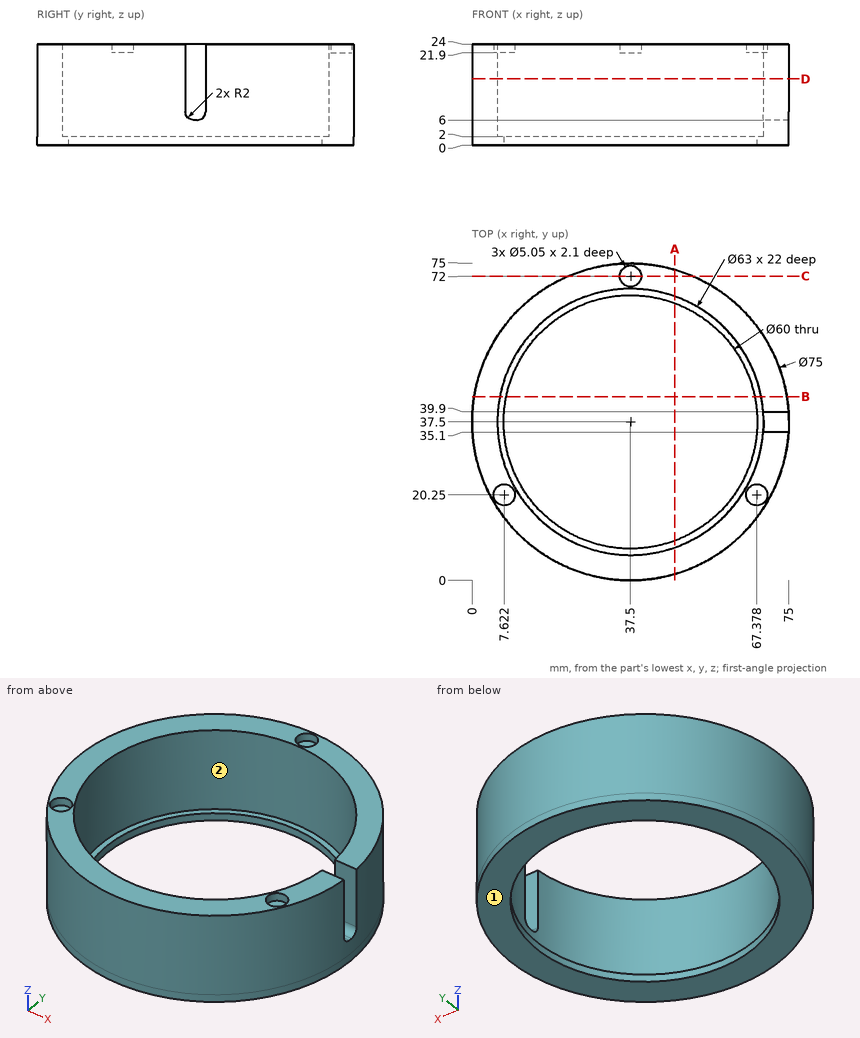
Could you check a few things on this drawing? It's one solid part, dimensions in mm from its lowest x, y, z. Coordinates: 2 decimals unless noted, no trailing zeros. Loops run counter-clockwise (first coordinate to the right, second up) from the corner with the lowest first, then second, coordinate; pieces in that order, holes last. Notation, with made-up numbers: (-30, 6) - (-18, 6) arc R32 cw to (-18, 37) - close; hole circle Ø2 at (11, 27.5). An arc over 180 degrees is marked (long way). Answer as a JSON object with one key per item and string values. Group by question number.
Item 1: If we section it at A-A (x = 48): List the corners of the cut face in (y, z) for me.
Item 2: If we mould it in two halves opening along Y, with no side actions, what happens to the marked faces 1 and 2? For each: released by +Y, released by -Y, zero draft, split by the parting line, or undercut.
Item 3: For pin 1 (0.9 mm diameter, centred on x = 72.5, y = 37.5, fed in from +Z); pin 2 (5 mm diameter, centred on x = 40.5, z = 14, fed in from -Y); pin 3 (6.5 mm diameter, centred on x = 73.5, z = 19, fed in from +Y); pin 4 (5 mm diameter, centred on x = 43.5, y = 12.5, fed in from -Z), each with a flat end and sliding along its axis, tell me the tip position at first contact or that it passes through.
Item 4: If we section it at D-D (z = 15.75): List the corners of the cut face in (x, y) for me, plus the area to 3 significant figures.
Item 5: If we section it at B-B (y = 43.5): List the corners of the cut face in (x, z) for me, plus the area to 3 significant figures.
Item 6: If I drill on L1, parallel to Y at x = 37.5, z = 17.5; L2, parallel to X at y = 20.25, z = 22.65; L3, parallel to Z at x = 66.5, y = 29.5, over which ranges is the centre line in solid material (lowest first)? Write a range as from..to.
Item 7: If we section it at C-C (y = 72): List the corners of the cut face in (x, z) for me (3 decimals).
Returned:
{
 "1": {"outline": "(1.5, 0) - (9.4, 0) - (9.4, 2) - (7.8, 2) - (7.8, 24) - (1.5, 24) - close; (65.6, 0) - (73.5, 0) - (73.5, 24) - (67.2, 24) - (67.2, 2) - (65.6, 2) - close"},
 "2": {"face 1": "zero draft", "face 2": "undercut"},
 "3": {"pin 1": "stops at z = 6", "pin 2": "stops at y = 0", "pin 3": "stops at y = 55.77", "pin 4": "passes through"},
 "4": {"outline": "(68.91, 35.1) arc R31.5 cw (long way) to (68.91, 39.9) - (74.92, 39.9) arc R37.5 ccw (long way) to (74.92, 35.1) - close", "area": "1,270 mm²"},
 "5": {"outline": "(0.48, 0) - (8.11, 0) - (8.11, 2) - (6.58, 2) - (6.58, 24) - (0.48, 24) - close; (66.89, 0) - (74.52, 0) - (74.52, 24) - (68.42, 24) - (68.42, 2) - (66.89, 2) - close", "area": "299 mm²"},
 "6": {"L1": "y = 0..6, 69..75", "L2": "x = 4.2..5.1, 10.15..11.14, 63.86..64.85, 69.9..70.8", "L3": "z = 0..2"},
 "7": {"outline": "(22.803, 0) - (52.197, 0) - (52.197, 24) - (40.025, 24) - (40.025, 21.9) - (34.975, 21.9) - (34.975, 24) - (22.803, 24) - close"}
}
